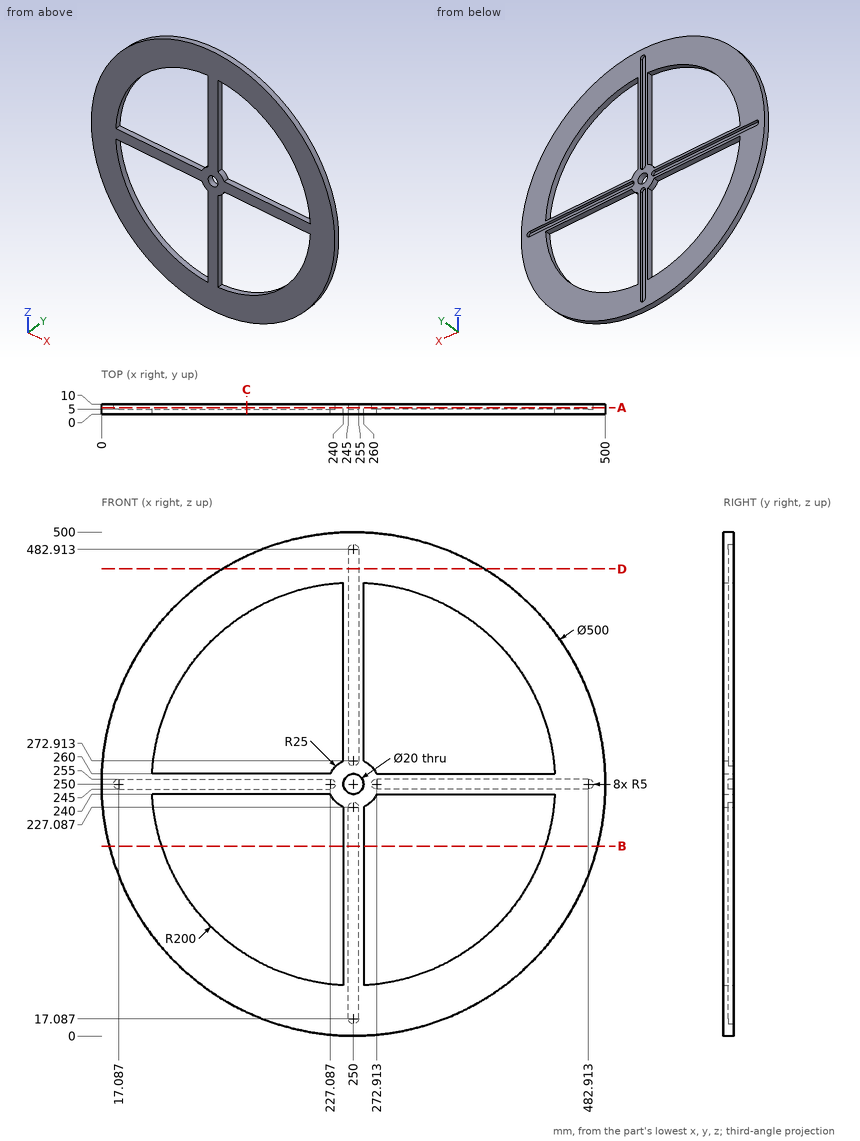
The drawing under review shows one solid part. Ordinate dimensions are in mm from its lowest x, y, z. Round coordinates to 2 decimals unless told otherwise and drop trailing zeros. Write each loop counter-clockwise with the first axis right and the second up, starting at its lowest first coordinate (ties: lowest second). Pieces come first, ordered by that corner, then holes.
(1) We need section B-B on z = 188.5. Give the boundary of the cut face in (x, y).
(2) We need section C-C on x = 144. Give the boundary of the cut face in (y, z), and give its area (3 significant figures).
(3) We need section A-A on y = 6.5. Give the number of separate pieces and of enclosed holes in the cut face, and give its area (3 significant figures).
(4) Wall thickness on L1, parallel to Z at x = 250, y = 6; L2, parallel to Z at x = 250, y = 3.25: over which ranges is each line inside the solid? List them lowest first.
(5) We need section D-D on z = 463.5. Give the boundary of the cut face in (x, y).
(6) Insertion check: pin 1 (5 mm diameter, centred on x = 203.5, y = 4, fed in from -Z); pin 2 (2.5 mm diameter, centred on x = 108.5, y = 7, fed in from -Z); pin 3 (5 mm diameter, centred on y = 5.5, z = 100, fed in from +X); pin 4 (16 mm diameter, centred on x = 250, z = 250, fed in from +Y). Each pin has a flat end and moves straight along its axis. Give the tip position at first contact, or say it passes through.
Findings below:
1. outline: (7.68, 0) - (59.69, 0) - (59.69, 10) - (7.68, 10) - close; (240, 0) - (260, 0) - (260, 10) - (255, 10) - (255, 5) - (245, 5) - (245, 10) - (240, 10) - close; (440.31, 0) - (492.32, 0) - (492.32, 10) - (440.31, 10) - close
2. outline: (0, 23.58) - (10, 23.58) - (10, 80.4) - (0, 80.4) - close; (0, 240) - (10, 240) - (10, 245) - (5, 245) - (5, 255) - (10, 255) - (10, 260) - (0, 260) - close; (0, 419.6) - (10, 419.6) - (10, 476.42) - (0, 476.42) - close
2. area: 1,290 mm2
3. separate pieces: 1
3. enclosed holes: 9
3. area: 77,700 mm2
4. L1: z = 0 to 12.09, 232.09 to 240, 260 to 267.91, 487.91 to 500
4. L2: z = 0 to 240, 260 to 500
5. outline: (119.93, 0) - (380.07, 0) - (380.07, 10) - (255, 10) - (255, 5) - (245, 5) - (245, 10) - (119.93, 10) - close
6. pin 1: stops at z = 3.9
6. pin 2: stops at z = 43.05
6. pin 3: stops at x = 451.85
6. pin 4: passes through
